The drawing under review shows one solid part. Ordinate dimensions are in mm from its lowest x, y, z. A direction names the side the tool comes from. Round coordinates to 2 decimals unless told otherwise and drop trailing zeros. Order: outer loops, then holes, each group sorted by start corner. A loop starts at its lowest first (then second) coordinate and runs counter-clockwise, first axis right, second up. Notation, with made-up numbers: M 27.25,-27 L 85.25,-27 A13 cw 85.25,-22 Z; hole C 79,74.5 d8. An arc over 180 degrees is marked long. Answer as a JSON object with one key per item and string values. Group by question number.
1) Consider section D-D, the plane x = 4.25. Write out the cut boundary in (y, z).
2) To check wall thickness, follow line 1 (X direction, y = 4.5, z = 8); line 2 (Y direction, x = 14.75, z = 6); line 3 (Y direction, x = 14, z = 6.25). State the ranges of each line that lie inside material, in increasing order.
3) For the marked faces 1, 2 and 3, list the 3-axis set-ups (+Z, -Z, +X, -X, +Y, -Y) from which the entire face can be reached by the end or side of a thin tool; tool diameter is ignored.
4) Consider section A-A, the plane y = 4. Write out the cut boundary in (x, z), then the cut area to 3 significant figures.
5) Consider section C-C, the plane z = 8.25. Write out the cut boundary in (x, y) (3 decimals).
6) Consider section B-B, the plane x = 13. Write out the cut boundary in (y, z), then the cut area to 3 significant figures.
7) The part is to be moulded in two halves that separate along Y. For the marked faces 4, 5 and 6, say which applies: +Y half, -Y half, draft (parallel to the pull), parting line (faces both ways), or undercut.
8) Insertion check: pin 1 Ø0.5 at (x, y) = (10, 5.5) entering from +Z; pin 2 Ø1.5 at (x, y) = (17, 5.5) entering from +Z. Each pin has a flat end and moves straight along its axis. Give the tip position at first contact, or say it passes through.
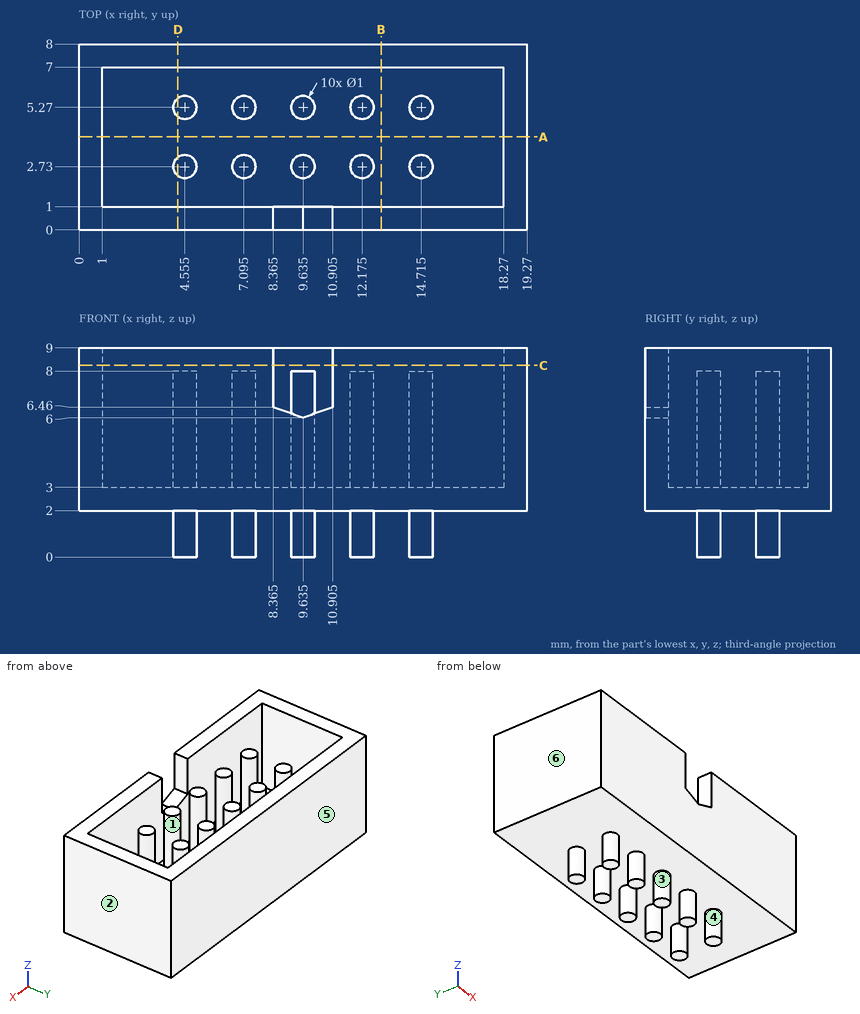
Results list:
{
 "1": {"outline": "M 0,2 L 2.33,2 L 2.33,0 L 3.13,0 L 3.13,2 L 4.87,2 L 4.87,0 L 5.67,0 L 5.67,2 L 8,2 L 8,9 L 7,9 L 7,3 L 5.67,3 L 5.67,8 L 4.87,8 L 4.87,3 L 3.13,3 L 3.13,8 L 2.33,8 L 2.33,3 L 1,3 L 1,9 L 0,9 Z"},
 "2": {"line 1": "0 to 1, 18.27 to 19.27", "line 2": "0 to 1, 2.23 to 3.23, 4.77 to 5.77, 7 to 8", "line 3": "0 to 1, 7 to 8"},
 "3": {"face 1": "+Z", "face 2": "+Z, -Z, +X, +Y, -Y", "face 3": "-Z"},
 "4": {"outline": "M 0,2 L 19.27,2 L 19.27,9 L 18.27,9 L 18.27,3 L 1,3 L 1,9 L 0,9 Z", "area": "31.3 mm^2"},
 "5": {"outline": "M 0,0 L 8.365,0 L 8.365,1 L 1,1 L 1,7 L 18.27,7 L 18.27,1 L 10.905,1 L 10.905,0 L 19.27,0 L 19.27,8 L 0,8 Z"},
 "6": {"outline": "M 0,2 L 8,2 L 8,9 L 7,9 L 7,3 L 1,3 L 1,9 L 0,9 Z", "area": "20.0 mm^2"},
 "7": {"face 4": "undercut", "face 5": "+Y half", "face 6": "draft"},
 "8": {"pin 1": "z = 8", "pin 2": "z = 3"}
}
